For this review, take the finished solid that the model builds, in its own axes (mm). A direction names the side the tool comes from. Give positions to 0.01 mm unless a question says otherwise; leave off trailing zeros. Put each result on its own line as item: value. Start each with the question number.
from build123d import *

# Parameters (mm, degrees)
SKETCH1_W                      = 57
SKETCH1_H                      = 42
BOSS_EXTRUDE1_DEPTH            = 8
BOSS_EXTRUDE2_DEPTH            = 397
SKETCH3_W                      = 72
SKETCH3_H                      = 56
BOSS_EXTRUDE3_DEPTH            = 8
SKETCH4_W                      = 55
SKETCH4_H                      = 56
BOSS_EXTRUDE4_DEPTH            = 54
CUT_EXTRUDE1_DEPTH             = 50
SKETCH6_R                      = 8
BOSS_EXTRUDE5_DEPTH            = 368.3
SKETCH7_W                      = 31.8
SKETCH7_H                      = 42
BOSS_EXTRUDE6_DEPTH            = 30
SKETCH8_R                      = 10
BOSS_EXTRUDE7_DEPTH            = 25
SKETCH9_R                      = 15
CUT_EXTRUDE2_DEPTH             = 5
BOSS_EXTRUDE8_REACH            = 67.7
SKETCH10_R                     = 3.175
SKETCH11_W                     = 4.3
SKETCH11_H                     = 397
CUT_EXTRUDE3_DEPTH             = 5.4
SKETCH12_W                     = 3.6
SKETCH12_H                     = 397
CUT_EXTRUDE4_DEPTH             = 2.7
SKETCH13_W                     = 4.3
SKETCH13_H                     = 397
CUT_EXTRUDE5_DEPTH             = 6.8
SKETCH14_W                     = 3.3
SKETCH14_H                     = 397
CUT_EXTRUDE6_DEPTH             = 3.4
M4X0_7_TAPPED_HOLE1_D          = 3.3
M4X0_7_TAPPED_HOLE1_DEPTH      = 10.1
M4X0_7_TAPPED_HOLE1_TIP        = 0.991420021
M4X0_7_TAPPED_HOLE2_AT_2_COUNT = 2
M4X0_7_TAPPED_HOLE2_AT_2_PITCH = 30
M4X0_7_TAPPED_HOLE2_AT_3_COUNT = 2
M4X0_7_TAPPED_HOLE2_AT_3_PITCH = 15.044018745
M4X0_7_TAPPED_HOLE2_AT_4_COUNT = 2
M4X0_7_TAPPED_HOLE2_AT_4_PITCH = 23.162955338
M5X0_8_TAPPED_HOLE1_AT_2_COUNT = 2
M5X0_8_TAPPED_HOLE1_AT_2_PITCH = 16.5


with BuildPart() as part:
    # Sketch1 → Boss-Extrude1 (new body)
    with BuildSketch(Plane(origin=(0, 0, 0), x_dir=(1, 0, 0), z_dir=(0, 1, 0))):
        with Locations((28.5, 0)):
            Rectangle(SKETCH1_W, SKETCH1_H)
    extrude(amount=BOSS_EXTRUDE1_DEPTH)

    # Sketch2 → Boss-Extrude2 (add)
    with BuildSketch(Plane(origin=(0, 8, 0), x_dir=(1, 0, 0), z_dir=(0, 1, 0))):
        Polygon((0, 21), (0, -21), (24.5, -21), (24.5, -14), (14.1, -14), (14.1, 14), (24.5, 14), (24.5, 21), align=None)
    extrude(amount=BOSS_EXTRUDE2_DEPTH)

    # Sketch3 → Boss-Extrude3 (add)
    with BuildSketch(Plane(origin=(0, 405, 0), x_dir=(1, 0, 0), z_dir=(0, 1, 0))):
        with Locations((36, 0)):
            Rectangle(SKETCH3_W, SKETCH3_H)
    extrude(amount=BOSS_EXTRUDE3_DEPTH)

    # Sketch4 → Boss-Extrude4 (add)
    with BuildSketch(Plane(origin=(0, 413, 0), x_dir=(1, 0, 0), z_dir=(0, 1, 0))):
        with Locations((44.5, 0)):
            Rectangle(SKETCH4_W, SKETCH4_H)
    extrude(amount=BOSS_EXTRUDE4_DEPTH)

    # Sketch5 → Cut-Extrude1 (cut)
    with BuildSketch(Plane(origin=(0, 467, 0), x_dir=(1, 0, 0), z_dir=(0, 1, 0))):
        with BuildLine():
            Line((17, 28), (17, 20.5))
            ThreePointArc((17, 20.5), (22.303300859, 22.696699141), (24.5, 28))
            Line((24.5, 28), (17, 28))
        make_face()
        with BuildLine():
            Line((72, 28), (64.5, 28))
            ThreePointArc((64.5, 28), (66.696699141, 22.696699141), (72, 20.5))
            Line((72, 20.5), (72, 28))
        make_face()
        with BuildLine():
            Line((72, -28), (72, -20.5))
            ThreePointArc((72, -20.5), (66.696699141, -22.696699141), (64.5, -28))
            Line((64.5, -28), (72, -28))
        make_face()
        with BuildLine():
            Line((17, -28), (24.5, -28))
            ThreePointArc((24.5, -28), (22.303300859, -22.696699141), (17, -20.5))
            Line((17, -20.5), (17, -28))
        make_face()
    extrude(amount=-CUT_EXTRUDE1_DEPTH, mode=Mode.SUBTRACT)

    # Sketch6 → Boss-Extrude5 (add)
    with BuildSketch(Plane(origin=(0, 8, 0), x_dir=(1, 0, 0), z_dir=(0, 1, 0))):
        with Locations((44.5, 0)):
            Circle(SKETCH6_R)
    extrude(amount=BOSS_EXTRUDE5_DEPTH)

    # Sketch7 → Boss-Extrude6 (add, symmetric)
    with BuildSketch(Plane(origin=(0, 338, 0), x_dir=(1, 0, 0), z_dir=(0, 1, 0))):
        with Locations((41.6, 0)):
            Rectangle(SKETCH7_W, SKETCH7_H)
    extrude(amount=BOSS_EXTRUDE6_DEPTH, both=True)

    # Sketch8 → Boss-Extrude7 (add)
    with BuildSketch(Plane(origin=(0, 376.3, 0), x_dir=(1, 0, 0), z_dir=(0, 1, 0))):
        with Locations((44.5, 0)):
            Circle(SKETCH8_R)
    extrude(amount=BOSS_EXTRUDE7_DEPTH)

    # Sketch9 → Cut-Extrude2 (cut)
    with BuildSketch(Plane.XZ.offset(-405)):
        with Locations((44.5, 0)):
            Circle(SKETCH9_R)
    extrude(amount=-CUT_EXTRUDE2_DEPTH, mode=Mode.SUBTRACT)

    # Sketch10 → Boss-Extrude8 (add, up to next)
    with BuildSketch(Plane(origin=(0, 401.3, 0), x_dir=(1, 0, 0), z_dir=(0, 1, 0)), mode=Mode.PRIVATE) as boss_extrude8_sk1:
        with Locations((44.5, 0)):
            Circle(SKETCH10_R)
    boss_extrude8_tool1 = extrude(boss_extrude8_sk1.sketch, amount=BOSS_EXTRUDE8_REACH, mode=Mode.PRIVATE) - part.part
    add(boss_extrude8_tool1.solids().sort_by_distance((44.5, 401.3, 0))[0])

    # Sketch11 → Cut-Extrude3 (cut)
    with BuildSketch(Plane(origin=(0, 0, -21), x_dir=(-1, 0, 0), z_dir=(0, 0, -1))):
        with Locations((-18.15, 206.5)):
            Rectangle(SKETCH11_W, SKETCH11_H)
    cut_extrude3 = extrude(amount=-CUT_EXTRUDE3_DEPTH, mode=Mode.SUBTRACT)

    # Sketch12 → Cut-Extrude4 (cut, symmetric)
    with BuildSketch(Plane(origin=(18.15, 0, 0), x_dir=(0, 0, -1), z_dir=(1, 0, 0))):
        with Locations((17.4, 206.5)):
            Rectangle(SKETCH12_W, SKETCH12_H)
    cut_extrude4 = extrude(amount=CUT_EXTRUDE4_DEPTH, both=True, mode=Mode.SUBTRACT)

    # Mirror1: Cut-Extrude3, Cut-Extrude4 across plane
    add(cut_extrude3.mirror(Plane.XY), mode=Mode.SUBTRACT)
    add(cut_extrude4.mirror(Plane.XY), mode=Mode.SUBTRACT)

    # Sketch13 → Cut-Extrude5 (cut)
    with BuildSketch(Plane.ZY):
        with Locations((15, 206.5)):
            Rectangle(SKETCH13_W, SKETCH13_H)
    cut_extrude5 = extrude(amount=-CUT_EXTRUDE5_DEPTH, mode=Mode.SUBTRACT)

    # Sketch14 → Cut-Extrude6 (cut, symmetric)
    with BuildSketch(Plane.XY.offset(15)):
        with Locations((3.65, 206.5)):
            Rectangle(SKETCH14_W, SKETCH14_H)
    cut_extrude6 = extrude(amount=CUT_EXTRUDE6_DEPTH, both=True, mode=Mode.SUBTRACT)

    # Mirror2: Cut-Extrude5, Cut-Extrude6 across plane
    add(cut_extrude5.mirror(Plane.XY), mode=Mode.SUBTRACT)
    add(cut_extrude6.mirror(Plane.XY), mode=Mode.SUBTRACT)

    # M4x0.7 Tapped Hole1
    with Locations(Plane(origin=(57.5, 0, 0), x_dir=(0, 0, -1), z_dir=(1, 0, 0))):
        with Locations((-15, 353), (15, 353), (15, 323), (-15, 323)):
            Hole(M4X0_7_TAPPED_HOLE1_D / 2, depth=M4X0_7_TAPPED_HOLE1_DEPTH)
            with Locations((0, 0, -(M4X0_7_TAPPED_HOLE1_DEPTH + M4X0_7_TAPPED_HOLE1_TIP / 2))):  # 118° drill point
                Cone(0, M4X0_7_TAPPED_HOLE1_D / 2, M4X0_7_TAPPED_HOLE1_TIP, mode=Mode.SUBTRACT)

    # Sketch23 → M4x0.7 Tapped Hole2 (revolve, cut)
    with BuildSketch(Plane(origin=(51.15, 323, 21), x_dir=(0, -1, 0), z_dir=(1, 0, 0))):
        Polygon((0, 0), (0, 6.991420021), (1.65, 6), (1.65, 0), align=None)
    m4x0_7_tapped_hole2 = revolve(axis=Axis((51.15, 323, 27.35), (0, 0, -1)), mode=Mode.SUBTRACT)

    # M4x0.7 Tapped Hole2 at 2: M4x0.7 Tapped Hole2 ×2
    with Locations(*[(0, i * M4X0_7_TAPPED_HOLE2_AT_2_PITCH, 0) for i in range(1, M4X0_7_TAPPED_HOLE2_AT_2_COUNT)]):
        add(m4x0_7_tapped_hole2, mode=Mode.SUBTRACT)

    # M4x0.7 Tapped Hole2 at 3: M4x0.7 Tapped Hole2 ×2
    with Locations(*[Vector(-0.07644234, 0.997074004, 0) * (i * M4X0_7_TAPPED_HOLE2_AT_3_PITCH) for i in range(1, M4X0_7_TAPPED_HOLE2_AT_3_COUNT)]):
        add(m4x0_7_tapped_hole2, mode=Mode.SUBTRACT)

    # M4x0.7 Tapped Hole2 at 4: M4x0.7 Tapped Hole2 ×2
    with Locations(*[Vector(-0.761992576, 0.647585758, 0) * (i * M4X0_7_TAPPED_HOLE2_AT_4_PITCH) for i in range(1, M4X0_7_TAPPED_HOLE2_AT_4_COUNT)]):
        add(m4x0_7_tapped_hole2, mode=Mode.SUBTRACT)

    # Sketch25 → M5x0.8 Tapped Hole1 (revolve, cut)
    with BuildSketch(Plane(origin=(32.5, 362.5, 21), x_dir=(0, -1, 0), z_dir=(1, 0, 0))):
        Polygon((0, 0), (0, 11.2618073), (2.1, 10), (2.1, 0), align=None)
    m5x0_8_tapped_hole1 = revolve(axis=Axis((32.5, 362.5, 27.35), (0, 0, -1)), mode=Mode.SUBTRACT)

    # M5x0.8 Tapped Hole1 at 2: M5x0.8 Tapped Hole1 ×2
    with Locations(*[(i * M5X0_8_TAPPED_HOLE1_AT_2_PITCH, 0, 0) for i in range(1, M5X0_8_TAPPED_HOLE1_AT_2_COUNT)]):
        add(m5x0_8_tapped_hole1, mode=Mode.SUBTRACT)

    # Mirror3: M5x0.8 Tapped Hole1, M4x0.7 Tapped Hole2 across plane
    add(m5x0_8_tapped_hole1.mirror(Plane.XY), mode=Mode.SUBTRACT)
    add(m4x0_7_tapped_hole2.mirror(Plane.XY), mode=Mode.SUBTRACT)

    # Mirror3 copy 1 sketch → Mirror3 copy 1 (revolve, cut)
    with BuildSketch(Plane(origin=(49, 362.5, -21), x_dir=(0, -1, 0), z_dir=(1, 0, 0))):
        Polygon((0, 0), (0, -11.2618073), (2.1, -10), (2.1, 0), align=None)
    revolve(axis=Axis((49, 362.5, -27.35), (0, 0, -1)), mode=Mode.SUBTRACT)

    # Mirror3 copy 2 sketch → Mirror3 copy 2 (revolve, cut)
    with BuildSketch(Plane(origin=(51.15, 353, -21), x_dir=(0, -1, 0), z_dir=(1, 0, 0))):
        Polygon((0, 0), (0, -6.991420021), (1.65, -6), (1.65, 0), align=None)
    revolve(axis=Axis((51.15, 353, -27.35), (0, 0, -1)), mode=Mode.SUBTRACT)

    # Mirror3 copy 3 sketch → Mirror3 copy 3 (revolve, cut)
    with BuildSketch(Plane(origin=(50, 338, -21), x_dir=(0, -1, 0), z_dir=(1, 0, 0))):
        Polygon((0, 0), (0, -6.991420021), (1.65, -6), (1.65, 0), align=None)
    revolve(axis=Axis((50, 338, -27.35), (0, 0, -1)), mode=Mode.SUBTRACT)

    # Mirror3 copy 4 sketch → Mirror3 copy 4 (revolve, cut)
    with BuildSketch(Plane(origin=(33.5, 338, -21), x_dir=(0, -1, 0), z_dir=(1, 0, 0))):
        Polygon((0, 0), (0, -6.991420021), (1.65, -6), (1.65, 0), align=None)
    revolve(axis=Axis((33.5, 338, -27.35), (0, 0, -1)), mode=Mode.SUBTRACT)


solid = part.part
1) Mouldability with a two-part tool opening along Z and no side actions: class faces 5 (the flat face through (38, 368, -5)), 6 (the flat face through (44, 410, 4)), 7 (the flat face through (14, 187, -21)) as released by +Z, released by -Z, zero draft, split by the parting line, or undercut.
2) Machinability: for faces 1 (the flat face through (57.5, 338, 0)), 2 (the flat face through (20, 417, 25)), 3 (the flat face through (35, 8, 0)), 4 (the flat face through (17, 440, 0)), which of the approach directions +Z, -Z, +X, -X, +Y, -Y give a long, thin tool a straight path to every point of the face, cutting with its end or side? Answer none if there is none.
3) Insertion check: P1, Ø16, axis at x = 47, z = 1.5, coming from the -Y side; P2, Ø5, axis at y = 279, z = -20, coming from the +X side; P3, Ø5, axis at x = 44, y = 116, coming from the +Z side; P4, Ø2.5, axis at y = 323, z = -15, coming from the -X side. Each pin has a flat end and moves straight along its axis. Give the tip position at first contact, or say it passes through.
4) Wall thickness on probe 1 along Y at (x, z) = (42, -8); probe 2 along X at (y, z) = (362.5, -18.5); probe 3 along X at (y, z) = (362.5, -12.75): over which ranges is each line inside the solid? List them lowest first.
Answers follow:
1. face 5: zero draft
1. face 6: undercut
1. face 7: released by -Z
2. face 1: +Z, -Z, +X, -Y
2. face 2: +Z, -X, +Y
2. face 3: none
2. face 4: +Z, -Z, -X, +Y
3. P1: y = 0
3. P2: x = 24.5
3. P3: z = 8
3. P4: x = 6.8
4. probe 1: 0 to 8, 308 to 368, 376.3 to 401.3, 410 to 467
4. probe 2: 0 to 15.45, 20.85 to 24.5, 25.7 to 30.4, 34.6 to 46.9, 51.1 to 57.5
4. probe 3: 0 to 2, 5.3 to 14.1, 25.7 to 30.4, 34.6 to 46.9, 51.1 to 57.5
